Answer from the drawing. Dimensions are ordinates in mm from the lowest x, y and z of the part. A direction names the side the tool comes from. Round coordinates to 2 decimals unless told otherwise and drop trailing zeros. Order: outer loops, then holes, each group sorted by start corner. A loop starts at its lowest first (then second) coordinate and runs counter-clockwise, first axis right, second up. Notation, with made-up numbers: (65.5, 18) -> (83.5, 18) arc R13 cw to (83.5, 31) -> close; hole circle Ø11 at (87.5, 17.25). An arc over 180 degrees is marked (long way). Use a Markdown table: item, result. Add a question column.
Item 1: A cutting plane is placed at B-B, the plane z = 3. Determine the outline of the cut face in (x, y).
Item 2: Find the intervals of material crossed by L1, parallel to X at y = 1.75, z = 3.5; L2, parallel to X at y = 1.5, z = 3; L3, parallel to Y at x = 5.5, z = 6.5, in increasing order. Write a range as [from, to].
Item 3: A cutting plane is placed at A-A, the plane x = 4. Determine the outline of the cut face in (y, z), plus the area to 3 significant figures.
Item 4: A cutting plane is placed at D-D, the plane y = 3.25. Determine the outline of the cut face in (x, z).
Item 5: A cutting plane is placed at C-C, the plane y = 8. Determine the outline of the cut face in (x, z).
Item 6: For a pull along X with two mould halves and no side action, classify the marked faces 3, 4 and 5 as +X half, -X half, draft (parallel to the pull), parting line (faces both ways), or undercut.
Item 7: Flat-ended cylindrical pins translate along their axes: P1, Ø1.5, axis at x = 5, y = 3, coming from the -Z side; P2, Ø1.5, axis at y = 5, z = 2.5, coming from the +X side; P3, Ø2.5, axis at x = 4, z = 3.46, coming from the -Y side; P4, Ø2, axis at y = 5, z = 2.5, coming from the +X side. Find the tip coordinate at first contact, or state that the pin passes through.
Item 8: A tool of negligible diameter and unlimited length cuts with its end or side. For the marked faces 1 and 2, from which of +Z, -Z, +X, -X, +Y, -Y can it reach the whole face along a straight path? Write none if from no direction.
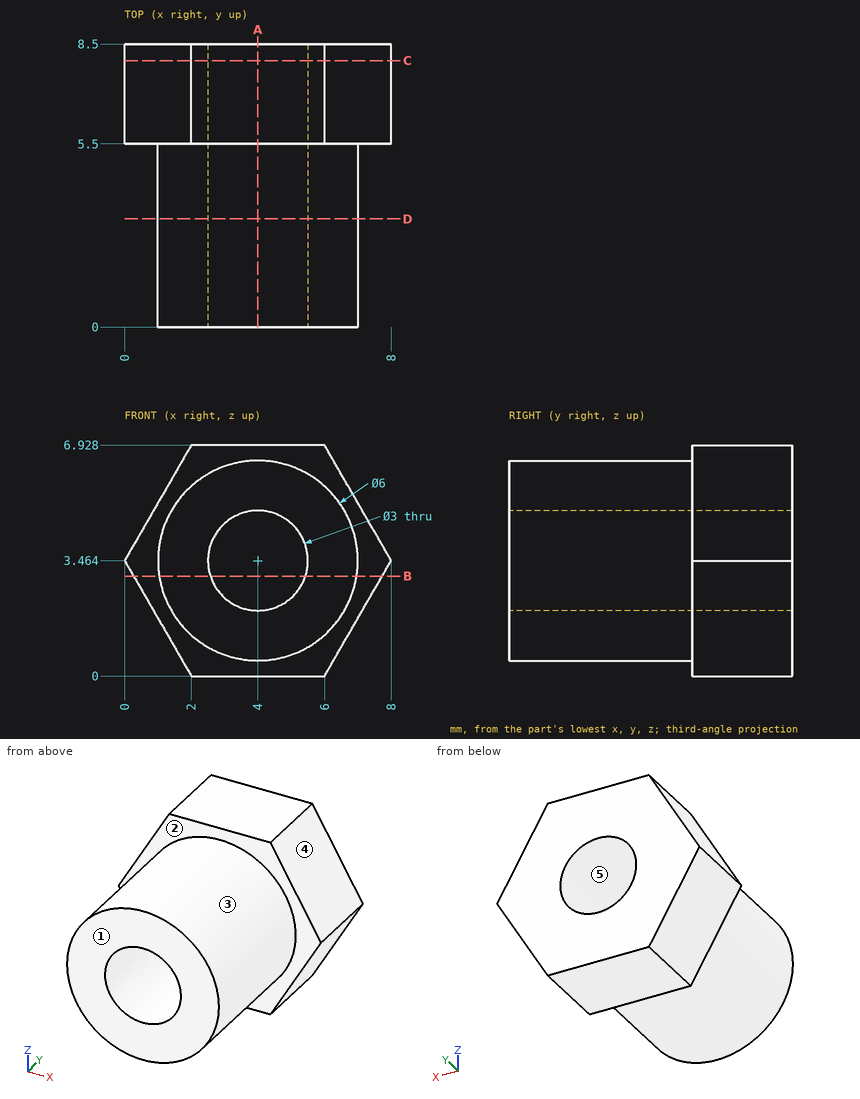
Reported:
| question | item | result |
|---|---|---|
| 1 | outline | (0.27, 5.5) -> (1.04, 5.5) -> (1.04, 0) -> (2.57, 0) -> (2.57, 8.5) -> (0.27, 8.5) -> close; (5.43, 0) -> (6.96, 0) -> (6.96, 5.5) -> (7.73, 5.5) -> (7.73, 8.5) -> (5.43, 8.5) -> close |
| 2 | L1 | [1, 2.5], [5.5, 7] |
| 2 | L2 | [1.04, 2.57], [5.43, 6.96] |
| 2 | L3 | [5.5, 8.5] |
| 3 | outline | (0, 0.46) -> (5.5, 0.46) -> (5.5, 0) -> (8.5, 0) -> (8.5, 1.96) -> (0, 1.96) -> close; (0, 4.96) -> (8.5, 4.96) -> (8.5, 6.93) -> (5.5, 6.93) -> (5.5, 6.46) -> (0, 6.46) -> close |
| 3 | area | 28.3 mm² |
| 4 | outline | circle Ø6 at (4, 3.46); hole circle Ø3 at (4, 3.46) |
| 5 | outline | (0, 3.46) -> (2, 0) -> (6, 0) -> (8, 3.46) -> (6, 6.93) -> (2, 6.93) -> close; hole circle Ø3 at (4, 3.46) |
| 6 | face 3 | parting line |
| 6 | face 4 | +X half |
| 6 | face 5 | undercut |
| 7 | P1 | z = 0.47 |
| 7 | P2 | x = 7.77 |
| 7 | P3 | through |
| 7 | P4 | x = 7.94 |
| 8 | face 1 | +Z, -Z, +X, -X, -Y |
| 8 | face 2 | -Y |
